CAD build for the part. Positions are in the model's coordinates, mm. Give positions to 0.01 mm unless a question says otherwise; leave off trailing zeros. Order: outer loops, then holes, each group sorted by start corner. A loop starts at its lowest first (then second) coordinate and runs counter-clockwise, first axis right, second up.
```python
from build123d import *

# Parameters (mm, degrees)
ESQUISSE1_R              = 7.5
ESQUISSE1_R_2            = 2.3
BOSS_EXTRU_1_DEPTH       = 6
ENL_V_MAT_EXTRU_9_DEPTH  = 10.5
ESQUISSE6_R              = 2.3
ENL_V_MAT_EXTRU_10_DEPTH = 50
ENL_V_MAT_EXTRU_11_DEPTH = 50
ESQUISSE9_R              = 2.5
ENL_V_MAT_EXTRU_12_DEPTH = 35
ESQUISSE3_R              = 2.3
ENL_V_MAT_EXTRU_13_DEPTH = 35
ESQUISSE10_R             = 2.3
ENL_V_MAT_EXTRU_14_DEPTH = 10


with BuildPart() as part:
    # Esquisse1 → Boss.-Extru.1 (new body)
    with BuildSketch(Plane(origin=(0, 0, 0), x_dir=(1, 0, 0), z_dir=(0, 1, 0))):
        Polygon((-150, 0), (-150, 260), (-110, 300), (110, 300), (150, 260), (150, 0), align=None)
        with Locations(Location((-120, 30, 0), (0, 0, 270))):
            Circle(ESQUISSE1_R, mode=Mode.SUBTRACT)
        with Locations(Location((-120, 267.5, 0), (0, 0, 270))):
            Circle(ESQUISSE1_R, mode=Mode.SUBTRACT)
        with Locations(Location((120, 268.5, 0), (0, 0, 270))):
            Circle(ESQUISSE1_R, mode=Mode.SUBTRACT)
        with Locations(Location((-111.514718626, 275.985281374, 0), (0, 0, 270))):
            Circle(ESQUISSE1_R_2, mode=Mode.SUBTRACT)
        with Locations(Location((-128.485281374, 259.014718626, 0), (0, 0, 270))):
            Circle(ESQUISSE1_R_2, mode=Mode.SUBTRACT)
        with Locations(Location((111.514718626, 276.985281374, 0), (0, 0, 270))):
            Circle(ESQUISSE1_R_2, mode=Mode.SUBTRACT)
        with Locations(Location((128.485281374, 260.014718626, 0), (0, 0, 270))):
            Circle(ESQUISSE1_R_2, mode=Mode.SUBTRACT)
        with Locations(Location((120, 30, 0), (0, 0, 270))):
            Circle(ESQUISSE1_R, mode=Mode.SUBTRACT)
        with Locations(Location((120, 42, 0), (0, 0, 270))):
            Circle(ESQUISSE1_R_2, mode=Mode.SUBTRACT)
        with Locations(Location((-120, 42, 0), (0, 0, 270))):
            Circle(ESQUISSE1_R_2, mode=Mode.SUBTRACT)
        with Locations(Location((-120, 18, 0), (0, 0, 270))):
            Circle(ESQUISSE1_R_2, mode=Mode.SUBTRACT)
        with Locations(Location((-132, 30, 0), (0, 0, 270))):
            Circle(ESQUISSE1_R_2, mode=Mode.SUBTRACT)
        with Locations(Location((-108, 30, 0), (0, 0, 270))):
            Circle(ESQUISSE1_R_2, mode=Mode.SUBTRACT)
        with Locations(Location((108, 30, 0), (0, 0, 270))):
            Circle(ESQUISSE1_R_2, mode=Mode.SUBTRACT)
        with Locations(Location((132, 30, 0), (0, 0, 270))):
            Circle(ESQUISSE1_R_2, mode=Mode.SUBTRACT)
        with Locations(Location((120, 18, 0), (0, 0, 270))):
            Circle(ESQUISSE1_R_2, mode=Mode.SUBTRACT)
    extrude(amount=BOSS_EXTRU_1_DEPTH)

    # Esquisse7 → Enl_v. mat.-Extru.9 (cut)
    with BuildSketch(Plane(origin=(0, 6, 0), x_dir=(1, 0, 0), z_dir=(0, 1, 0))):
        Polygon((-130, 150), (-130, 182), (-140, 182), (-140, 118), (-130, 118), align=None)
    enl_v_mat_extru_9 = extrude(amount=-ENL_V_MAT_EXTRU_9_DEPTH, mode=Mode.SUBTRACT)

    # Esquisse6 → Enl_v. mat.-Extru.10 (cut)
    with BuildSketch(Plane(origin=(0, 6, 0), x_dir=(1, 0, 0), z_dir=(0, 1, 0))):
        with Locations(Location((-138.5, 90, 0), (0, 0, 270))):
            Circle(ESQUISSE6_R)
        with Locations(Location((-138.5, 112, 0), (0, 0, 270))):
            Circle(ESQUISSE6_R)
        with Locations(Location((-106.5, 112, 0), (0, 0, 270))):
            Circle(ESQUISSE6_R)
        with Locations(Location((-106.5, 90, 0), (0, 0, 270))):
            Circle(ESQUISSE6_R)
    enl_v_mat_extru_10 = extrude(amount=-ENL_V_MAT_EXTRU_10_DEPTH, mode=Mode.SUBTRACT)

    # Esquisse4 → Enl_v. mat.-Extru.11 (cut)
    with BuildSketch(Plane(origin=(0, 6, 0), x_dir=(1, 0, 0), z_dir=(0, 1, 0))):
        Polygon((-100, 150), (-100, 182), (-64, 182), (-64, 118), (-100, 118), align=None)
    enl_v_mat_extru_11 = extrude(amount=-ENL_V_MAT_EXTRU_11_DEPTH, mode=Mode.SUBTRACT)

    # Sym_trie1: Enl_v. mat.-Extru.9 across plane
    add(enl_v_mat_extru_9.mirror(Plane(origin=(0, 0, 0), x_dir=(0, 0, 1), z_dir=(1, 0, 0))), mode=Mode.SUBTRACT)

    # Sym_trie2: Enl_v. mat.-Extru.11 across plane
    add(enl_v_mat_extru_11.mirror(Plane(origin=(0, 0, 0), x_dir=(0, 0, 1), z_dir=(1, 0, 0))), mode=Mode.SUBTRACT)

    # Sym_trie3: Enl_v. mat.-Extru.10 across plane
    add(enl_v_mat_extru_10.mirror(Plane(origin=(0, 0, 0), x_dir=(0, 0, 1), z_dir=(1, 0, 0))), mode=Mode.SUBTRACT)

    # Esquisse9 → Enl_v. mat.-Extru.12 (cut)
    with BuildSketch(Plane(origin=(0, 6, 0), x_dir=(1, 0, 0), z_dir=(0, 1, 0))):
        with Locations(Location((-100, 50, 0), (0, 0, 270))):
            Circle(ESQUISSE9_R)
        with Locations(Location((100, 50, 0), (0, 0, 270))):
            Circle(ESQUISSE9_R)
        with Locations(Location((100, 250, 0), (0, 0, 270))):
            Circle(ESQUISSE9_R)
        with Locations(Location((-100, 250, 0), (0, 0, 270))):
            Circle(ESQUISSE9_R)
    extrude(amount=-ENL_V_MAT_EXTRU_12_DEPTH, mode=Mode.SUBTRACT)

    # Esquisse3 → Enl_v. mat.-Extru.13 (cut)
    with BuildSketch(Plane(origin=(0, 6, 0), x_dir=(1, 0, 0), z_dir=(0, 1, 0))):
        with Locations(Location((-60, 174, 0), (0, 0, 270))):
            Circle(ESQUISSE3_R)
        with Locations(Location((-60, 116, 0), (0, 0, 270))):
            Circle(ESQUISSE3_R)
        with Locations(Location((-30, 166, 0), (0, 0, 270))):
            Circle(ESQUISSE3_R)
        with Locations(Location((-30, 124, 0), (0, 0, 270))):
            Circle(ESQUISSE3_R)
        with Locations(Location((60, 184, 0), (0, 0, 270))):
            Circle(ESQUISSE3_R)
        with Locations(Location((30, 176, 0), (0, 0, 270))):
            Circle(ESQUISSE3_R)
        with Locations(Location((30, 134, 0), (0, 0, 270))):
            Circle(ESQUISSE3_R)
        with Locations(Location((60, 126, 0), (0, 0, 270))):
            Circle(ESQUISSE3_R)
    extrude(amount=-ENL_V_MAT_EXTRU_13_DEPTH, mode=Mode.SUBTRACT)

    # Esquisse10 → Enl_v. mat.-Extru.14 (cut)
    with BuildSketch(Plane(origin=(0, 6, 0), x_dir=(1, 0, 0), z_dir=(0, 1, 0))):
        with Locations(Location((-19, 73, 0), (0, 0, 270))):
            Circle(ESQUISSE10_R)
        with Locations(Location((-19, 117, 0), (0, 0, 270))):
            Circle(ESQUISSE10_R)
        with Locations(Location((25, 73, 0), (0, 0, 270))):
            Circle(ESQUISSE10_R)
        with Locations(Location((25, 117, 0), (0, 0, 270))):
            Circle(ESQUISSE10_R)
        with Locations(Location((-24.999750468, 227, 0), (0, 0, 270))):
            Circle(ESQUISSE10_R)
        with Locations(Location((-24.999750468, 183, 0), (0, 0, 270))):
            Circle(ESQUISSE10_R)
        with Locations(Location((19, 183, 0), (0, 0, 270))):
            Circle(ESQUISSE10_R)
        with Locations(Location((19, 227, 0), (0, 0, 270))):
            Circle(ESQUISSE10_R)
    extrude(amount=-ENL_V_MAT_EXTRU_14_DEPTH, mode=Mode.SUBTRACT)


solid = part.part
```
Item 1: Wall check: L1, parallel to X at y = 1.4, z = -50; L2, parallel to X at y = 4.85, z = -112; L3, parallel to X at y = 4.95, z = -250.5. Give the ranges that are in metal, low to high.
Item 2: Slice it at A-A (x = 91). Give the cut face in (y, z).
Item 3: Two-plate mould, pull along Z, no slides. Class faces 1 (the face through (2, 6, -152)), 2 (the face through (112.68, 2.96, -31.63)), 3 (the face through (-130, 3, -280)): released by +Z, released by -Z, zero draft, split by the parting line, or undercut.
Item 4: Slice it at B-B (z = -267.5). Give the cut face in (x, y).
Item 5: Slice it at C-C (y = 2.2). State how many separate pieces and enclosed holes the cut face has, and give its area (3 significant figures).
A:
1. L1: x = -150 to -102.5, -97.5 to 97.5, 102.5 to 150
1. L2: x = -150 to -140.8, -136.2 to -108.8, -104.2 to 104.2, 108.8 to 136.2, 140.8 to 150
1. L3: x = -150 to -102.45, -97.55 to 97.55, 102.45 to 150
2. outline: (0, -300) - (6, -300) - (6, -182) - (0, -182) - close; (0, -118) - (6, -118) - (6, 0) - (0, 0) - close
3. face 1: zero draft
3. face 2: undercut
3. face 3: released by -Z
4. outline: (-142.5, 0) - (-127.5, 0) - (-127.5, 6) - (-142.5, 6) - close; (-112.5, 0) - (112.57, 0) - (112.57, 6) - (-112.5, 6) - close; (127.43, 0) - (142.5, 0) - (142.5, 6) - (127.43, 6) - close
5. separate pieces: 1
5. enclosed holes: 48
5. area: 81,100 mm2
